```python
from build123d import *

# Parameters (mm, degrees)
IZIM1_R                     = 50
Y_KSEKLIK_EKSTR_ZYON1_DEPTH = 2
KES_EKSTR_ZYON2_DEPTH       = 2
DAIRESEL_KAPLAMA2_COUNT     = 23
IZIM12_R                    = 40
Y_KSEKLIK_EKSTR_ZYON2_DEPTH = 3
Y_KSEKLIK_EKSTR_ZYON3_START = -3
IZIM13_R                    = 40
Y_KSEKLIK_EKSTR_ZYON3_DEPTH = 3
IZIM14_R                    = 12
KES_EKSTR_ZYON6_DEPTH       = 7
DAIRESEL_KAPLAMA5_COUNT     = 5
KES_EKSTR_ZYON7_DEPTH       = 7


with BuildPart() as part:
    # Çizim1 → Yükseklik-Ekstrüzyon1 (new body)
    with BuildSketch(Plane(origin=(0, 0, 0), x_dir=(1, 0, 0), z_dir=(0, 1, 0))):
        with Locations(Location((0, 0, 0), (0, 0, 270))):
            Circle(IZIM1_R)
    extrude(amount=Y_KSEKLIK_EKSTR_ZYON1_DEPTH)

    # Çizim2 → Kes-Ekstrüzyon2 (cut)
    with BuildSketch(Plane(origin=(0, 2, 0), x_dir=(1, 0, 0), z_dir=(0, 1, 0))):
        with BuildLine():
            Line((-7.668264722, 58.995898097), (5.736778926, 51.800614184))
            Line((5.736778926, 51.800614184), (4.056392608, 45.540740741))
            ThreePointArc((4.056392608, 45.540740741), (0, 42.42962963), (-4.056392608, 45.540740741))
            Line((-4.056392608, 45.540740741), (-7.668264722, 58.995898097))
        make_face()
    kes_ekstr_zyon2 = extrude(amount=-KES_EKSTR_ZYON2_DEPTH, mode=Mode.SUBTRACT)

    # Dairesel Kaplama2: Kes-Ekstrüzyon2 ×23 about axis
    dairesel_kaplama2_axis = Axis((0, 0, 0), (0, 1, 0))
    for i in range(1, DAIRESEL_KAPLAMA2_COUNT):
        add(kes_ekstr_zyon2.rotate(dairesel_kaplama2_axis, i * 360 / DAIRESEL_KAPLAMA2_COUNT), mode=Mode.SUBTRACT)

    # Çizim12 → Yükseklik-Ekstrüzyon2 (add)
    with BuildSketch(Plane(origin=(0, 2, 0), x_dir=(1, 0, 0), z_dir=(0, 1, 0))):
        with Locations(Location((0, 0, 0), (0, 0, 270))):
            Circle(IZIM12_R)
    extrude(amount=Y_KSEKLIK_EKSTR_ZYON2_DEPTH)

    # Çizim13 → Yükseklik-Ekstrüzyon3 (add)
    with BuildSketch(Plane(origin=(0, 0, 0), x_dir=(1, 0, 0), z_dir=(0, 1, 0)).offset(Y_KSEKLIK_EKSTR_ZYON3_START)):
        with Locations(Location((0, 0, 0), (0, 0, 270))):
            Circle(IZIM13_R)
    extrude(amount=Y_KSEKLIK_EKSTR_ZYON3_DEPTH)

    # Çizim14 → Kes-Ekstrüzyon6 (cut, symmetric)
    with BuildSketch(Plane(origin=(0, 2, 0), x_dir=(1, 0, 0), z_dir=(0, 1, 0))):
        with Locations(Location((-17.67766953, 17.67766953, 0), (0, 0, 270))):
            Circle(IZIM14_R)
    kes_ekstr_zyon6 = extrude(amount=KES_EKSTR_ZYON6_DEPTH, both=True, mode=Mode.SUBTRACT)

    # Dairesel Kaplama5: Kes-Ekstrüzyon6 ×5 about axis
    dairesel_kaplama5_axis = Axis((0, 0, 0), (0, 1, 0))
    for i in range(1, DAIRESEL_KAPLAMA5_COUNT):
        add(kes_ekstr_zyon6.rotate(dairesel_kaplama5_axis, i * 360 / DAIRESEL_KAPLAMA5_COUNT), mode=Mode.SUBTRACT)

    # Çizim16 → Kes-Ekstrüzyon7 (cut, symmetric)
    with BuildSketch(Plane(origin=(0, 2, 0), x_dir=(1, 0, 0), z_dir=(0, 1, 0))):
        with BuildLine():
            Line((-4.609772229, 3), (4.609772229, 3))
            ThreePointArc((4.609772229, 3), (0, -5.5), (-4.609772229, 3))
        make_face()
    extrude(amount=KES_EKSTR_ZYON7_DEPTH, both=True, mode=Mode.SUBTRACT)


solid = part.part
```
Geometry: final body of the model. Coordinates: model frame, mm. A direction names the side the tool comes from. Coordinates: 2 decimals unless noted, no trailing zeros. Use CSV: the item, a comma, the result in double quotes.
1) Access query for faces 1 (the flat face through (-28.675, 1.014, -38.28)), 2 (the flat face through (23.196, 1.014, 41.828)), 3 (the flat face through (-43.314, 1.014, 20.287)). Directions: +Z, -Z, +X, -X, +Y, -Y. A direction counts if a zero-diameter tool reaches every point of the face in a straight line with its end or side. Return the directions, or none.
Findings:
face 1,"-Z, +Y, -Y"
face 2,"+Z, +Y, -Y"
face 3,"-X, +Y, -Y"
2) Mould query, pull axis X, two halves, no side actions, for faces 4 (the flat face through (-31.68, 1.01, -35.92)), 5 (the flat face through (34, 0, -22)), 6 (the cylindrical face through (-30.957, 1.014, -29.017)), 7 (the cylindrical face through (42.326, 1.014, 2.972)). Classes: +X half, -X half, draft (parallel to the pull), parting line (faces both ways), or undercut.
Findings:
face 4,"-X half"
face 5,"draft"
face 6,"undercut"
face 7,"+X half"
3) Line query: line 1 (Z direction, x = 21.5, y = -2.25); line 2 (Z direction, x = -14.5, y = 2.25); line 3 (X direction, y = -0.5, z = -26). Output: solid intervals per line, ascending.
Findings:
line 1,"z = -33.73 to -28.68, -15.87 to -7.66, 15.48 to 33.73"
line 2,"z = -37.28 to -29.25, -6.11 to 2.21, 20.49 to 37.28"
line 3,"x = -30.4 to -26.32, -9.03 to -0.06, 22.76 to 30.4"
4) Pin query (flat end, axial travel): pin 1 Ø2 at (y, z) = (3.5, -31) entering from -X; pin 2 Ø4 at (x, y) = (21.5, 1) entering from +Z; pin 3 Ø1.5 at (y, z) = (3.5, -15) entering from -X. Return the tip coordinate at first contact, or that it passes through.
Findings:
pin 1,"stops at x = -26.46"
pin 2,"stops at z = 42.21"
pin 3,"stops at x = -37.38"
